The model under review builds one solid part; all positions refer to its coordinate system, in mm. A direction names the side the tool comes from. Coordinates: 2 decimals unless noted, no trailing zeros. Write each loop counter-clockwise with the first axis right and the second up, starting at its lowest first coordinate (ties: lowest second). Pieces come first, ordered by that corner, then holes.
```python
from build123d import *

# Parameters (mm, degrees)
ESQUISSE1_R             = 2.5
BOSS_EXTRU_1_DEPTH      = 18.5
ENL_V_MAT_EXTRU_1_DEPTH = 6


with BuildPart() as part:
    # Esquisse1 → Boss.-Extru.1 (new body)
    with BuildSketch(Plane.XY):
        Circle(ESQUISSE1_R)
    extrude(amount=BOSS_EXTRU_1_DEPTH)

    # Esquisse2 → Enlèv. mat.-Extru.1 (cut)
    with BuildSketch(Plane.XY):
        with BuildLine():
            Line((-2, 1.5), (2, 1.5))
            ThreePointArc((2, 1.5), (0, 2.5), (-2, 1.5))
        make_face()
        with BuildLine():
            Line((-2, -1.5), (2, -1.5))
            ThreePointArc((2, -1.5), (0, -2.5), (-2, -1.5))
        make_face()
    extrude(amount=ENL_V_MAT_EXTRU_1_DEPTH, mode=Mode.SUBTRACT)


solid = part.part
```
Item 1: To check wall thickness, follow line 1 along Z through (x, y) = (-1, -1.65); line 2 along Y through (x, z) = (-0.7, 1.25); line 3 along X through (y, z) = (-1.1, 15.25) (3 decimals). State the ranges of each line that lie inside material, in increasing order.
Solved:
line 1: z = 6 to 18.5
line 2: y = -1.5 to 1.5
line 3: x = -2.245 to 2.245
Item 2: Take a section at D-D, the plane y = 0.5. Write out the cut boundary in (x, z), plus the area to 3 significant figures.
Solved:
outline: (-2.45, 0) - (2.45, 0) - (2.45, 18.5) - (-2.45, 18.5) - close
area: 90.6 mm2
Item 3: Take a section at C-C, the plane x = 0. Write out the cut boundary in (y, z), plus the area to 3 significant figures.
Solved:
outline: (-2.5, 6) - (-1.5, 6) - (-1.5, 0) - (1.5, 0) - (1.5, 6) - (2.5, 6) - (2.5, 18.5) - (-2.5, 18.5) - close
area: 80.5 mm2
Item 4: Take a section at A-A, the plane x = 1.5. Write out the cut boundary in (y, z).
Solved:
outline: (-2, 6) - (-1.5, 6) - (-1.5, 0) - (1.5, 0) - (1.5, 6) - (2, 6) - (2, 18.5) - (-2, 18.5) - close
Item 5: Machinability: for faces 1 (the face through (0, 0, 18.5)), 2 (the face through (0, 1.5, 3)), 3 (the face through (0, -1.5, 3)), which of the approach directions +Z, -Z, +X, -X, +Y, -Y give a long, thin tool a straight path to every point of the face, cutting with its end or side? Answer none if there is none.
Solved:
face 1: +Z, +X, -X, +Y, -Y
face 2: -Z, +X, -X, +Y
face 3: -Z, +X, -X, -Y
Item 6: Take a section at B-B, the plane z = 10.25. Write out the cut boundary in (x, y), plus the area to 3 significant figures.
Solved:
outline: circle Ø5 at (0, 0)
area: 19.6 mm2
Item 7: For pin 1 (1.5 mm diameter, centred on x = 1.5, z = 15.5, fed in from +Y); pin 2 (3 mm diameter, centred on x = -0.5, z = 2.5, fed in from -Y), all flat-tipped, find the tip position at first contact; note any pin that passes through.
Solved:
pin 1: stops at y = 2.38
pin 2: stops at y = -1.5
